Print and shaded views of the part. All mm, measured from the part's lowest x, y and z. Coordinates: 2 decimals unless noted, no trailing zeros. Loops run counter-clockwise (first coordinate to the right, second up) from the corner with the lowest first, then second, coordinate; pieces in that order, holes last. Notation, with made-up numbers: M 33.25,25.5 L 60.25,25.5 A28 cw 60.25,60.5 Z; hole C -31.75,-19 d4. An arc over 180 degrees is marked long. One line per question, with ' | ' between items. Start each with the question number.
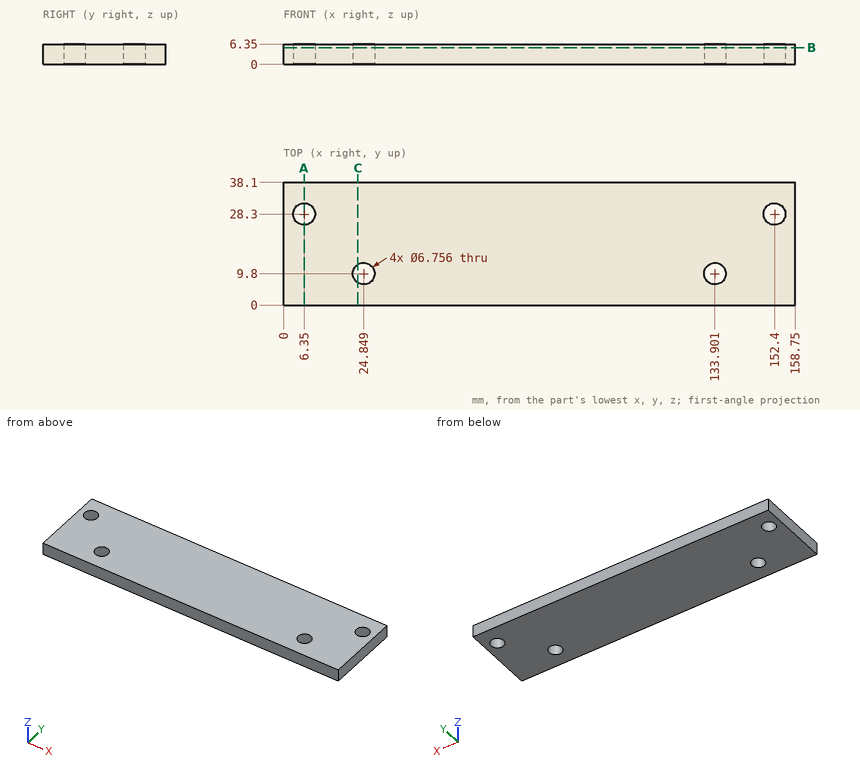
(1) Band-saw the part on A-A on x = 6.35. Write the cut outline in (y, z).
(2) Band-saw the part on C-C on x = 23. Write the cut outline in (y, z), then the cut area to 3 significant figures.
(3) Pin check, flat tips, straight feed: P1, Ø5, axis at x = 49.5, y = 5.5, coming from the -Z side; P2, Ø4, axis at x = 6.35, y = 28.3, coming from the -Z side. Stop position of each tip, or through.
(4) Drill centre lines: line 1 (Y direction, x = 134, z = 4); line 2 (X direction, y = 8, z = 4.25); line 3 (Y direction, x = 152.4, z = 4.25). Where is each one in solid material? Low to high. Write a range as [from, to].
(5) Band-saw the part on B-B on z = 5.25. Write the cut outline in (x, y).
Computed values:
1) outline: M 0,0 L 24.92,0 L 24.92,6.35 L 0,6.35 Z; M 31.68,0 L 38.1,0 L 38.1,6.35 L 31.68,6.35 Z
2) outline: M 0,0 L 6.97,0 L 6.97,6.35 L 0,6.35 Z; M 12.63,0 L 38.1,0 L 38.1,6.35 L 12.63,6.35 Z | area: 206 mm^2
3) P1: z = 0 | P2: through
4) line 1: [0, 6.42], [13.18, 38.1] | line 2: [0, 21.99], [27.71, 131.04], [136.76, 158.75] | line 3: [0, 24.92], [31.68, 38.1]
5) outline: M 0,0 L 158.75,0 L 158.75,38.1 L 0,38.1 Z; hole C 6.35,28.3 d6.76; hole C 24.85,9.8 d6.76; hole C 133.9,9.8 d6.76; hole C 152.4,28.3 d6.76
